Part model, mm, in its own coordinate system. Face numbers are marked on the shaded views. A direction names the side the tool comes from. Give positions to 0.01 mm unless a question says otherwise; leave off trailing zeros. Write each loop counter-clockwise with the first axis right and the second up, starting at its lowest first coordinate (ties: lowest second). Pieces come first, ordered by that corner, then holes. Notation, with made-up numbers: M -28.75,-27 L 19.25,-27 A20 cw 19.25,-12 Z; hole C 75.25,0 d7. An arc over 180 degrees is marked long. Answer as CSV lines item,"result". Start each with the question number.
Item 1: Band-saw the part on D-D, the plane x = 72. List the corners of the cut face in (y, z).
Item 2: Two-plate mould, pull along X, no slides. Class the marked faces 1, 2, 3 and 4: +X half, -X half, draft (parallel to the pull), parting line (faces both ways), or undercut.
Item 3: Wall check: L1, parallel to Z at x = -38.1, y = 119.5; L2, parallel to Z at x = -162.5, y = 7; L3, parallel to X at y = 124.5, z = -32.5. Give the ranges that are in metal, low to high. Write a range as from..to.
Item 4: 3-axis set-ups, long thin cutter, end or side, ignore diameter. For the marked faces 5, 6, 7, 8 and 9: which of +Z, -Z, +X, -X, +Y, -Y reach the whole face in a straight line?
Item 5: Band-saw the part on C-C, the plane z = 3.5. List the corners of the cut face in (x, y).
Item 6: Pin check, flat tips, straight feed: pin 1 (7.5 mm diameter, centred on x = 38.1, z = -39.69, fed in from -Y); pin 2 (9.5 mm diameter, centred on y = 99, z = -28.5, fed in from +X); pin 3 (9.5 mm diameter, centred on x = 160, y = 94, fed in from +Z); pin 4 (4 mm diameter, centred on y = 34.92, z = 33.34, fed in from -X). Stop position of each tip, or through.
Item 7: Band-saw the part on B-B, the plane z = 50.5. List the corners of the cut face in (x, y), then the cut area to 3 significant figures.
Item 8: Band-saw the part on A-A, the plane x = 151. List the corners of the cut face in (y, z), then the cut area to 3 significant figures.
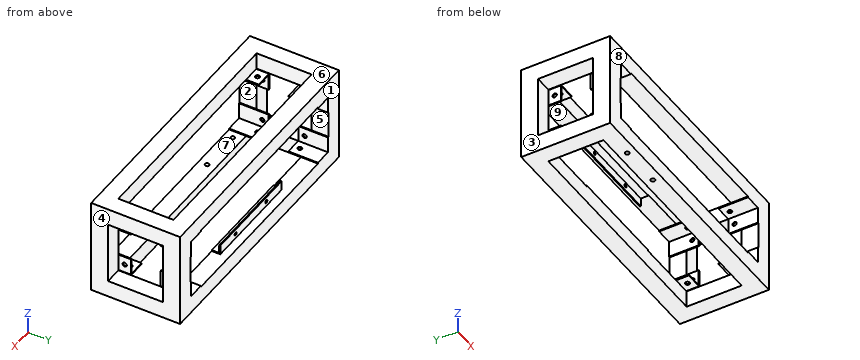
from build123d import *

# Parameters (mm, degrees)
SKETCH1_W            = 393.7
SKETCH1_H            = 144.4625
BOSS_EXTRUDE1_DEPTH  = 133.35
SKETCH6_W            = 342.9
SKETCH6_H            = 82.55
CUT_EXTRUDE4_DEPTH   = 279.211356537
SKETCH7_W            = 93.6625
SKETCH7_H            = 82.55
CUT_EXTRUDE5_DEPTH   = 422.899592292
SKETCH8_W            = 342.9
SKETCH8_H            = 93.6625
CUT_EXTRUDE6_DEPTH   = 249.494463674
SKETCH10_W           = 25.4
SKETCH10_H           = 44.45
SKETCH10_R           = 3.175
BOSS_EXTRUDE7_DEPTH  = 1.5875
SKETCH12_W           = 25.4
SKETCH12_H           = 44.45
SKETCH12_R           = 3.175
BOSS_EXTRUDE8_DEPTH  = 1.5875
SKETCH13_W           = 152.4
SKETCH13_H           = 12.7
BOSS_EXTRUDE9_DEPTH  = 1.5875
SKETCH14_W           = 152.4
SKETCH14_H           = 1.5875
BOSS_EXTRUDE10_DEPTH = 12.7
CUT_EXTRUDE8_REACH   = 243.917
SKETCH15_R           = 2.38125
CUT_EXTRUDE10_REACH  = 280.211
SKETCH17_R           = 3.175


with BuildPart() as part:
    # Sketch1 → Boss-Extrude1 (new body)
    with BuildSketch(Plane(origin=(0, 0, 0), x_dir=(1, 0, 0), z_dir=(0, 1, 0))):
        Rectangle(SKETCH1_W, SKETCH1_H)
    extrude(amount=BOSS_EXTRUDE1_DEPTH)

    # Sketch6 → Cut-Extrude4 (cut, through all)
    with BuildSketch(Plane.XY.offset(72.23125)):
        with Locations((0, 66.675)):
            Rectangle(SKETCH6_W, SKETCH6_H)
    extrude(amount=-CUT_EXTRUDE4_DEPTH, mode=Mode.SUBTRACT)

    # Sketch7 → Cut-Extrude5 (cut, through all)
    with BuildSketch(Plane.ZY.offset(196.85)):
        with Locations((0, 66.675)):
            Rectangle(SKETCH7_W, SKETCH7_H)
    extrude(amount=-CUT_EXTRUDE5_DEPTH, mode=Mode.SUBTRACT)

    # Sketch8 → Cut-Extrude6 (cut, through all)
    with BuildSketch(Plane(origin=(0, 133.35, 0), x_dir=(1, 0, 0), z_dir=(0, 1, 0))):
        Rectangle(SKETCH8_W, SKETCH8_H)
    extrude(amount=-CUT_EXTRUDE6_DEPTH, mode=Mode.SUBTRACT)

    # Sketch10 → Boss-Extrude7 (add)
    # profile 1 of 4: a face of its own
    with BuildSketch(Plane(origin=(0, 0, 46.83125), x_dir=(-1, 0, 0), z_dir=(0, 0, -1))):
        with Locations((-157.95625, 22.225)):
            Rectangle(SKETCH10_W, SKETCH10_H)
        with Locations((-157.95625, 34.925)):
            Circle(SKETCH10_R, mode=Mode.SUBTRACT)
    # profile 2 of 4: a face of its own
    with BuildSketch(Plane(origin=(0, 0, 46.83125), x_dir=(-1, 0, 0), z_dir=(0, 0, -1))):
        with Locations((157.95625, 22.225)):
            Rectangle(SKETCH10_W, SKETCH10_H)
        with Locations(Location((157.95625, 34.925, 0), (0, 0, 180))):
            Circle(SKETCH10_R, mode=Mode.SUBTRACT)
    # profile 3 of 4: a face of its own
    with BuildSketch(Plane(origin=(0, 0, 46.83125), x_dir=(-1, 0, 0), z_dir=(0, 0, -1))):
        with Locations((157.95625, 111.125)):
            Rectangle(SKETCH10_W, SKETCH10_H)
        with Locations((157.95625, 98.425)):
            Circle(SKETCH10_R, mode=Mode.SUBTRACT)
    # profile 4 of 4: a face of its own
    with BuildSketch(Plane(origin=(0, 0, 46.83125), x_dir=(-1, 0, 0), z_dir=(0, 0, -1))):
        with Locations((-157.95625, 111.125)):
            Rectangle(SKETCH10_W, SKETCH10_H)
        with Locations(Location((-157.95625, 98.425, 0), (0, 0, 180))):
            Circle(SKETCH10_R, mode=Mode.SUBTRACT)
    boss_extrude7 = extrude(amount=BOSS_EXTRUDE7_DEPTH)

    # Mirror5: Boss-Extrude7 across plane
    add(boss_extrude7.mirror(Plane.XY))

    # Sketch12 → Boss-Extrude8 (add)
    # profile 1 of 4: a face of its own
    with BuildSketch(Plane.ZY.offset(-171.45)):
        with Locations((-33.3375, 22.225)):
            Rectangle(SKETCH12_W, SKETCH12_H)
        with Locations((-33.3375, 34.925)):
            Circle(SKETCH12_R, mode=Mode.SUBTRACT)
    # profile 2 of 4: a face of its own
    with BuildSketch(Plane.ZY.offset(-171.45)):
        with Locations((33.3375, 22.225)):
            Rectangle(SKETCH12_W, SKETCH12_H)
        with Locations(Location((33.3375, 34.925, 0), (0, 0, 180))):
            Circle(SKETCH12_R, mode=Mode.SUBTRACT)
    # profile 3 of 4: a face of its own
    with BuildSketch(Plane.ZY.offset(-171.45)):
        with Locations((33.3375, 111.125)):
            Rectangle(SKETCH12_W, SKETCH12_H)
        with Locations((33.3375, 98.425)):
            Circle(SKETCH12_R, mode=Mode.SUBTRACT)
    # profile 4 of 4: a face of its own
    with BuildSketch(Plane.ZY.offset(-171.45)):
        with Locations((-33.3375, 111.125)):
            Rectangle(SKETCH12_W, SKETCH12_H)
        with Locations(Location((-33.3375, 98.425, 0), (0, 0, 180))):
            Circle(SKETCH12_R, mode=Mode.SUBTRACT)
    boss_extrude8 = extrude(amount=BOSS_EXTRUDE8_DEPTH)

    # Mirror6: Boss-Extrude8 across plane
    add(boss_extrude8.mirror(Plane(origin=(0, 0, 0), x_dir=(0, 0, 1), z_dir=(1, 0, 0))))

    # Sketch13 → Boss-Extrude9 (add)
    with BuildSketch(Plane(origin=(0, 0, 46.83125), x_dir=(-1, 0, 0), z_dir=(0, 0, -1))):
        with Locations((0, 114.3)):
            Rectangle(SKETCH13_W, SKETCH13_H)
    boss_extrude9 = extrude(amount=BOSS_EXTRUDE9_DEPTH)

    # Sketch14 → Boss-Extrude10 (add)
    with BuildSketch(Plane(origin=(0, 0, 45.24375), x_dir=(-1, 0, 0), z_dir=(0, 0, -1))):
        with Locations((0, 119.85625)):
            Rectangle(SKETCH14_W, SKETCH14_H)
    boss_extrude10 = extrude(amount=BOSS_EXTRUDE10_DEPTH)

    # Sketch15 → Cut-Extrude8 (cut, up to next)
    with BuildSketch(Plane(origin=(0, 120.65, 0), x_dir=(1, 0, 0), z_dir=(0, 1, 0)), mode=Mode.PRIVATE) as cut_extrude8_sk1:
        with Locations(Location((-38.1, -39.6875, 0), (0, 0, 180))):
            Circle(SKETCH15_R)
    cut_extrude8_tool1 = extrude(cut_extrude8_sk1.sketch, amount=-CUT_EXTRUDE8_REACH, mode=Mode.PRIVATE) & part.part
    # Sketch15 → Cut-Extrude8 (cut, up to next)
    with BuildSketch(Plane(origin=(0, 120.65, 0), x_dir=(1, 0, 0), z_dir=(0, 1, 0)), mode=Mode.PRIVATE) as cut_extrude8_sk2:
        with Locations(Location((38.1, -39.6875, 0), (0, 0, 270))):
            Circle(SKETCH15_R)
    cut_extrude8_tool2 = extrude(cut_extrude8_sk2.sketch, amount=-CUT_EXTRUDE8_REACH, mode=Mode.PRIVATE) & part.part
    cut_extrude8_1 = cut_extrude8_tool1.solids().sort_by_distance((-38.1, 120.65, 39.6875))[0]
    add(cut_extrude8_1, mode=Mode.SUBTRACT)
    cut_extrude8_2 = cut_extrude8_tool2.solids().sort_by_distance((38.1, 120.65, 39.6875))[0]
    add(cut_extrude8_2, mode=Mode.SUBTRACT)
    cut_extrude8 = cut_extrude8_1 + cut_extrude8_2  # Cut-Extrude8 as one shape, for the pattern or mirror that repeats it

    # Mirror7: Boss-Extrude9, Boss-Extrude10, Cut-Extrude8 across plane
    add(boss_extrude9.mirror(Plane.XY))
    add(boss_extrude10.mirror(Plane.XY))
    add(cut_extrude8.mirror(Plane.XY), mode=Mode.SUBTRACT)

    # Sketch17 → Cut-Extrude10 (cut, up to next)
    with BuildSketch(Plane(origin=(0, 0, -72.23125), x_dir=(-1, 0, 0), z_dir=(0, 0, -1)), mode=Mode.PRIVATE) as cut_extrude10_sk1:
        with Locations((69.85, 12.7)):
            Circle(SKETCH17_R)
    cut_extrude10_tool1 = extrude(cut_extrude10_sk1.sketch, amount=-CUT_EXTRUDE10_REACH, mode=Mode.PRIVATE) & part.part
    # Sketch17 → Cut-Extrude10 (cut, up to next)
    with BuildSketch(Plane(origin=(0, 0, -72.23125), x_dir=(-1, 0, 0), z_dir=(0, 0, -1)), mode=Mode.PRIVATE) as cut_extrude10_sk2:
        with Locations((133.35, 12.7)):
            Circle(SKETCH17_R)
    cut_extrude10_tool2 = extrude(cut_extrude10_sk2.sketch, amount=-CUT_EXTRUDE10_REACH, mode=Mode.PRIVATE) & part.part
    add(cut_extrude10_tool1.solids().sort_by_distance((-69.85, 12.7, -72.23125))[0], mode=Mode.SUBTRACT)
    add(cut_extrude10_tool2.solids().sort_by_distance((-133.35, 12.7, -72.23125))[0], mode=Mode.SUBTRACT)


solid = part.part
Output:
1,outline,"M 0,-72.23 L 25.4,-72.23 L 25.4,-46.83 L 0,-46.83 Z; M 0,46.83 L 25.4,46.83 L 25.4,72.23 L 0,72.23 Z; M 107.95,-72.23 L 133.35,-72.23 L 133.35,-46.83 L 120.65,-46.83 L 120.65,-32.54 L 119.06,-32.54 L 119.06,-45.24 L 107.95,-45.24 Z; M 107.95,45.24 L 119.06,45.24 L 119.06,32.54 L 120.65,32.54 L 120.65,46.83 L 133.35,46.83 L 133.35,72.23 L 107.95,72.23 Z"
2,face 1,"draft"
2,face 2,"undercut"
2,face 3,"-X half"
2,face 4,"+X half"
3,L1,"-72.23..-42.07, -37.31..-32.54, 32.54..37.31, 42.07..72.23"
3,L2,"-72.23..-45.24, 45.24..72.23"
3,L3,"-196.85..-169.86, 169.86..196.85"
4,face 5,"+Y, -Y"
4,face 6,"+Z, +X, -X, +Y, -Y"
4,face 7,"-Y"
4,face 8,"+Z, -Z, +X, -X, -Y"
4,face 9,"+Y"
5,outline,"M -196.85,0 L -171.45,0 L -171.45,25.4 L -196.85,25.4 Z; M -196.85,107.95 L -171.45,107.95 L -171.45,133.35 L -196.85,133.35 Z; M 171.45,0 L 196.85,0 L 196.85,25.4 L 171.45,25.4 Z; M 171.45,107.95 L 196.85,107.95 L 196.85,133.35 L 171.45,133.35 Z"
6,pin 1,"y = 119.06"
6,pin 2,"x = 171.45"
6,pin 3,"z = 46.83"
6,pin 4,"through"
7,outline,"M -196.85,0 L 196.85,0 L 196.85,133.35 L -196.85,133.35 Z; hole M -171.45,25.4 L 171.45,25.4 L 171.45,107.95 L -171.45,107.95 Z"
7,area,"24,200 mm²"
8,outline,"M 0,-72.23 L 25.4,-72.23 L 25.4,-46.83 L 44.45,-46.83 L 44.45,-45.24 L 0,-45.24 Z; M 0,45.24 L 44.45,45.24 L 44.45,46.83 L 25.4,46.83 L 25.4,72.23 L 0,72.23 Z; M 88.9,-46.83 L 107.95,-46.83 L 107.95,-72.23 L 133.35,-72.23 L 133.35,-45.24 L 88.9,-45.24 Z; M 88.9,45.24 L 133.35,45.24 L 133.35,72.23 L 107.95,72.23 L 107.95,46.83 L 88.9,46.83 Z"
8,area,"2,860 mm²"
